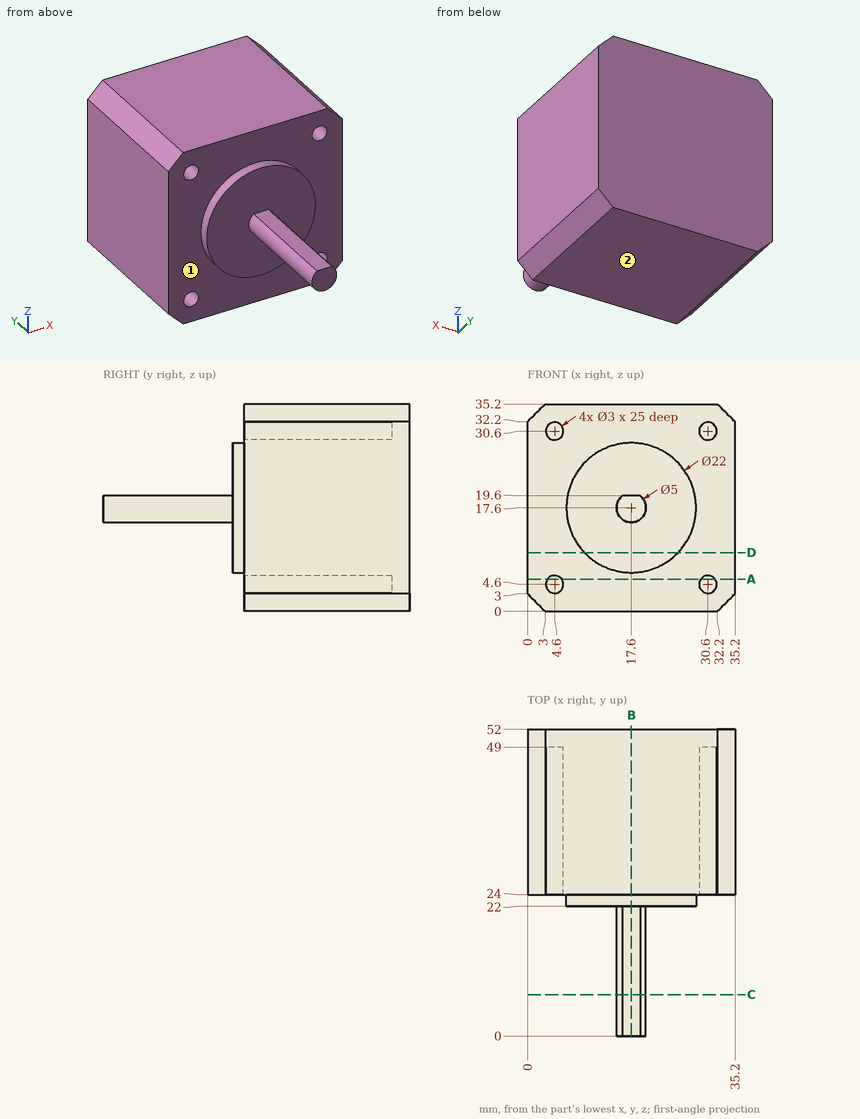
Part print with two shaded views. Sizes in mm from the minimum x, y, z corner. A direction names the side the tool comes from. Round coordinates to 2 decimals unless told otherwise and drop trailing zeros. Loops run counter-clockwise (first coordinate to the right, second up) from the corner with the lowest first, then second, coordinate; pieces in that order, holes last. Notation, with made-up numbers: (-2, -30) - (30, -30) arc R21 ccw to (30, 8) - close; hole circle Ø7 at (-38.5, -24). An arc over 180 degrees is marked (long way). Answer as a JSON object with one key per item and string values.
Item 1: Band-saw the part on A-A on z = 5.5. List the corners of the cut face in (x, y).
Output:
{"outline": "(0, 24) - (3.4, 24) - (3.4, 49) - (5.8, 49) - (5.8, 24) - (29.4, 24) - (29.4, 49) - (31.8, 49) - (31.8, 24) - (35.2, 24) - (35.2, 52) - (0, 52) - close"}
Item 2: Pin check, flat tips, straight feed: pin 1 (0.9 mm diameter, centred on x = 18.5, y = 11.5, fed in from +Z); pin 2 (12 mm diameter, centred on x = 11, z = 25, fed in from -Y); pin 3 (0.9 mm diameter, centred on x = 30, z = 4.5, fed in from -Y). Stop position of each tip, or through.
Output:
{"pin 1": "z = 19.6", "pin 2": "y = 22", "pin 3": "y = 49"}
Item 3: Band-saw the part on C-C on y = 7. List the corners of the cut face in (x, z), plus the area to 3 significant figures.
Output:
{"outline": "(16.1, 19.6) arc R2.5 ccw (long way) to (19.1, 19.6) - close", "area": "18.6 mm2"}
Item 4: Tool access for the marked faces 1 and 2: list every direction of +Z, -Z, +X, -X, +Y, -Y with a clear straight run to the whole face (end or side of a thin tool).
Output:
{"face 1": "-Y", "face 2": "-Z, +X, -X, +Y, -Y"}
Item 5: Wall check: L1, parallel to Z at x = 30.5, y = 41; L2, parallel to X at y = 42, z = 4; L3, parallel to X at y = 41.5, z = 5.5. Give the ranges that are in metal, low to high.
Output:
{"L1": "0 to 3.1, 6.1 to 29.1, 32.1 to 35.2", "L2": "0 to 3.23, 5.97 to 29.23, 31.97 to 35.2", "L3": "0 to 3.4, 5.8 to 29.4, 31.8 to 35.2"}
Item 6: Band-saw the part on D-D on z = 10. List the corners of the cut face in (x, y).
Output:
{"outline": "(0, 24) - (9.65, 24) - (9.65, 22) - (25.55, 22) - (25.55, 24) - (35.2, 24) - (35.2, 52) - (0, 52) - close"}
Item 7: Band-saw the part on B-B on x = 17.6. List the corners of the cut face in (y, z).
Output:
{"outline": "(0, 15.1) - (22, 15.1) - (22, 6.6) - (24, 6.6) - (24, 0) - (52, 0) - (52, 35.2) - (24, 35.2) - (24, 28.6) - (22, 28.6) - (22, 19.6) - (0, 19.6) - close"}
